```python
from build123d import *

# Parameters (mm, degrees)
BOSS_EXTRUDE2_DEPTH = 6
SKETCH4_R           = 0.85
CUT_EXTRUDE1_DEPTH  = 6
SKETCH6_R           = 0.85
CUT_EXTRUDE2_DEPTH  = 6


with BuildPart() as part:
    # Sketch3 → Boss-Extrude2 (new body)
    with BuildSketch(Plane.XY):
        Polygon((0, 0), (10, 0), (10, 1), (1, 1), (1, 8.5), (0, 8.5), align=None)
    extrude(amount=BOSS_EXTRUDE2_DEPTH)

    # Sketch4 → Cut-Extrude1 (cut)
    with BuildSketch(Plane(origin=(1, 0, 0), x_dir=(0, 0, -1), z_dir=(1, 0, 0))):
        with Locations(Location((-3, 5.5, 0), (0, 0, 90))):
            Circle(SKETCH4_R)
    extrude(amount=-CUT_EXTRUDE1_DEPTH, mode=Mode.SUBTRACT)

    # Sketch6 → Cut-Extrude2 (cut)
    with BuildSketch(Plane(origin=(0, 1, 0), x_dir=(1, 0, 0), z_dir=(0, 1, 0))):
        with Locations(Location((3, -3, 0), (0, 0, 180))):
            Circle(SKETCH6_R)
        with Locations(Location((8, -3, 0), (0, 0, 180))):
            Circle(SKETCH6_R)
    extrude(amount=-CUT_EXTRUDE2_DEPTH, mode=Mode.SUBTRACT)


solid = part.part
```
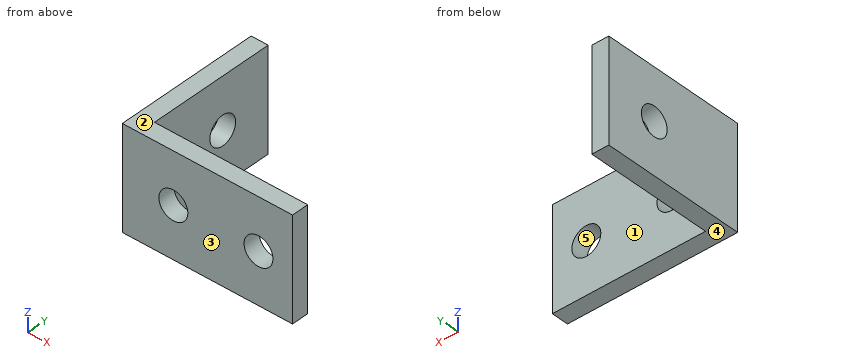
Part model, mm, in its own coordinate system. Face numbers are marked on the shaded views. A direction names the side the tool comes from. Coordinates: 2 decimals unless noted, no trailing zeros. Loops run counter-clockwise (first coordinate to the right, second up) from the corner with the lowest first, then second, coordinate; pieces in that order, holes last. Notation, with made-up numbers: (-17, 71.25) - (40, 71.25) arc R29 cw to (40, 104.25) - close; hole circle Ø1 at (12.25, 5.5). An arc over 180 degrees is marked (long way). Write item = value, one per line. Start each with the question number.
Item 1: Cut at B-B, the plane z = 3. Give the cut face in (x, y).
Item 2: Flat gauge pins, fed straight in: pin 1 Ø1.4 at (y, z) = (5.5, 3) entering from +X; pin 2 Ø3 at (x, z) = (5, 2) entering from +Y; pin 3 Ø1.8 at (y, z) = (4.5, 4) entering from +X. Where does each tip first touch, or does it go through?
Item 3: 3-axis set-ups, long thin cutter, end or side, ignore diameter. For the marked faces 1 and 2: which of +Z, -Z, +X, -X, +Y, -Y reach the whole face in a straight line?
Item 4: Mould opens along Z. For the marked faces 3, 4 and 5 say: released by +Z, released by -Z, zero draft, split by the parting line, or undercut.
Item 5: Cut at D-D, the plane z = 0.75. Give the cut face in (x, y), and give its area (3 significant figures).
Item 6: Cut at A-A, the plane x = 8. Give the cut face in (y, z).
Item 7: Wall check: L1, parallel to Z at x = 0.55, y = 5.5; L2, parallel to X at y = 4, z = 2.8. Give the ranges that are in metal, low to high. Write a range as from..to.
The answers:
q1.outline = (0, 0) - (2.15, 0) - (2.15, 1) - (1, 1) - (1, 4.65) - (0, 4.65) - close; (0, 6.35) - (1, 6.35) - (1, 8.5) - (0, 8.5) - close; (3.85, 0) - (7.15, 0) - (7.15, 1) - (3.85, 1) - close; (8.85, 0) - (10, 0) - (10, 1) - (8.85, 1) - close
q2.pin_1 = through
q2.pin_2 = 1
q2.pin_3 = 1
q3.face_1 = +Z, -Z, +X, +Y
q3.face_2 = +Z, +X, -X, +Y, -Y
q4.face_3 = zero draft
q4.face_4 = released by -Z
q4.face_5 = undercut
q5.outline = (0, 0) - (10, 0) - (10, 1) - (1, 1) - (1, 8.5) - (0, 8.5) - close
q5.area = 17.5 mm2
q6.outline = (0, 0) - (1, 0) - (1, 2.15) - (0, 2.15) - close; (0, 3.85) - (1, 3.85) - (1, 6) - (0, 6) - close
q7.L1 = 0..2.15, 3.85..6
q7.L2 = 0..1
